Input: part model. Units: mm. Frame: model coordinates. A direction names the side the tool comes from. Round coordinates to 2 decimals unless told otherwise and drop trailing zeros. Loops run counter-clockwise (first coordinate to the right, second up) from the corner with the lowest first, then second, coordinate; pieces in that order, holes last. Notation, with made-up numbers: M -12,-30.75 L 11,-30.75 A24 cw 11,-16.75 Z; hole C 42.25,89.5 d4. An arc over 180 degrees is marked long. Return JSON: item names as keys, results as strings. Group by question number.
1) Access query for faces 4 (the face through (64, -48, 11)), 5 (the face through (-75, 70, 10)), 6 (the face through (49, 67, -35)). Directions: +Z, -Z, +X, -X, +Y, -Y. A direction counts if a zero-diameter tool reaches every point of the face in a straight line with its end or side. Return the directions, or none.
2) Material intervals for line 1 (Z direction, x = -55, y = 29); line 2 (Y direction, x = 4.5, z = 3); line 3 (X direction, y = 22, z = 21.5), sorted ascending. Write a range as from..to.
3) Section C-C (z = -18.5). Output: boundary loops of the cut face in (x, y), plus the area to 3 significant figures.
4) Section A-A (x = -7). Output: boundary loops of the cut face in (y, z).
5) Contact query for flat-ended pins moving along their axis: P1, Ø7, axis at x = -103.5, z = 13.5, coming from the +Y side; P2, Ø3, axis at x = 11, z = 14.5, coming from the +Y side; P3, Ø9, axis at x = -46, y = 83.48, coming from the -Z side. Output: stop coordinate, or through.
6) Section B-B (y = 21.5). Output: boundary loops of the cut face in (x, z), plus the area to 3 significant figures.
7) Section D-D (y = 0). Output: boundary loops of the cut face in (x, z), plus the area to 3 significant figures.
8) Mould query, pull axis X, two halves, no side actions, for faces 1 (the face through (42, 63, -39)), 2 (the face through (69.983, 1.539, 9.86)), 3 (the face through (20.19, 77.41, 11.34)). Classes: +X half, -X half, draft (parallel to the pull), parting line (faces both ways), or undercut.
from build123d import *

# Parameters (mm, degrees)
SKETCH_R        = 60
PAD_DEPTH       = 23
POCKET_DEPTH    = 20
SKETCH002_R     = 10
PAD001_DEPTH    = 62
SKETCH005_R     = 2.8
POCKET001_DEPTH = 62.001
SKETCH006_R     = 5
POCKET002_DEPTH = 4
FILLET_R        = 16
FILLET001_R     = 18
FILLET002_R     = 2
FILLET003_R     = 1
SKETCH007_R     = 5
POCKET003_DEPTH = 15


with BuildPart() as part:
    # Sketch → Pad (new body)
    with BuildSketch(Plane.XY):
        with BuildLine():
            ThreePointArc((-78.765475, -14), (61.318839, -51.38093), (0, 80))
            Line((-150, 80), (0, 80))
            Line((-150, 80), (-150, 23.233627))
            Line((-150, 23.233627), (-78.765475, -14))
        make_face()
        Circle(SKETCH_R, mode=Mode.SUBTRACT)
    extrude(amount=PAD_DEPTH)

    # Sketch001 (on Face6 of Pad) → Pocket (cut)
    with BuildSketch(Plane(origin=(0, 0, 0), x_dir=(1, 0, 0), z_dir=(0, 0, -1))):
        with BuildLine():
            Line((-178.35, 70), (0, 70))
            ThreePointArc((0, -70), (70, 0), (0, 70))
            Line((-178.35, -70), (0, -70))
            Line((-178.35, 70), (-178.35, -70))
        make_face()
    extrude(amount=-POCKET_DEPTH, mode=Mode.SUBTRACT)

    # Sketch002 (on Face6 of Pocket) → Pad001 (join)
    with BuildSketch(Plane.XY.offset(23)):
        with Locations((47.02282, 64.72136)):
            Circle(SKETCH002_R)
        with Locations((-46.056914, 83.088872)):
            Circle(SKETCH002_R)
    extrude(amount=-PAD001_DEPTH)

    # Sketch005 (on Face5 of Pad001) → Pocket001 (cut, through all)
    with BuildSketch(Plane.XY.offset(23)):
        with Locations((-46.002335, 83.480621)):
            Circle(SKETCH005_R)
        with Locations((47.02282, 64.72136)):
            Circle(SKETCH005_R)
    extrude(amount=-POCKET001_DEPTH, mode=Mode.SUBTRACT)

    # Sketch006 (on Face12 of Pocket001) → Pocket002 (cut)
    with BuildSketch(Plane(origin=(0, 0, -39), x_dir=(1, 0, 0), z_dir=(0, 0, -1))):
        with Locations((-46.002335, -83.480621)):
            Circle(SKETCH006_R)
        with Locations((47.02282, -64.72136)):
            Circle(SKETCH006_R)
    extrude(amount=-POCKET002_DEPTH, mode=Mode.SUBTRACT)

    # Fillet
    fillet_edges = [part.edges().sort_by_distance(p)[0] for p in [
        (-78.765475, -14, 21.5),
    ]]
    fillet(fillet_edges, radius=FILLET_R)

    # Fillet001
    fillet001_edges = [part.edges().sort_by_distance(p)[0] for p in [
        (-150, 23.233627, 21.5),
    ]]
    fillet(fillet001_edges, radius=FILLET001_R)

    # Fillet002
    fillet002_edges = [part.edges().sort_by_distance(p)[0] for p in [
        (-150, 70, 10),
        (-150, 80, 11.5),
    ]]
    fillet(fillet002_edges, radius=FILLET002_R)

    # Fillet003
    fillet003_edges = [part.edges().sort_by_distance(p)[0] for p in [
        (-38.729833, -70, 10),
    ]]
    fillet(fillet003_edges, radius=FILLET003_R)

    # Sketch007 (on Face10 of Fillet003) → Pocket003 (cut)
    with BuildSketch(Plane.XY.offset(23)):
        with Locations((47.02282, 64.72136)):
            Circle(SKETCH007_R)
        with Locations((-46.002335, 83.480621)):
            Circle(SKETCH007_R)
    extrude(amount=-POCKET003_DEPTH, mode=Mode.SUBTRACT)


solid = part.part
Returned:
{
 "1": {"face 4": "+Z, -Z", "face 5": "-Z, -X", "face 6": "-Z"},
 "2": {"line 1": "z = 20..23", "line 2": "y = -79.87..-69.86, 69.86..79.87", "line 3": "x = -145.29..-55.82, 55.82..76.92"},
 "3": {"outline": "C -46.06,83.09 d20; C 47.02,64.72 d20; hole C -46,83.48 d5.6; hole C 47.02,64.72 d5.6", "area": "579 mm^2"},
 "4": {"outline": "M -79.69,0 L -70,0 L -70,20 L -59.59,20 L -59.59,23 L -79.69,23 Z; M 59.59,20 L 70,20 L 70,0 L 80,0 L 80,23 L 59.59,23 Z"},
 "5": {"P1": "stops at y = 80", "P2": "stops at y = 79.43", "P3": "stops at z = -35"},
 "6": {"outline": "M -144.82,20 L -56.02,20 L -56.02,23 L -144.82,23 Z; M 56.02,20 L 66.62,20 L 66.62,0 L 77.06,0 L 77.06,23 L 56.02,23 Z", "area": "538 mm^2"},
 "7": {"outline": "M -105.55,20 L -60,20 L -60,23 L -105.55,23 Z; M 60,20 L 70,20 L 70,0 L 80,0 L 80,23 L 60,23 Z", "area": "397 mm^2"},
 "8": {"face 1": "draft", "face 2": "-X half", "face 3": "undercut"}
}
